Can you work these out from the model? Positions are in its coordinate system, mm. Give positions to 0.01 mm unless a question says otherwise; leave off trailing zeros. Answer as a JSON object with one key per item and string values.
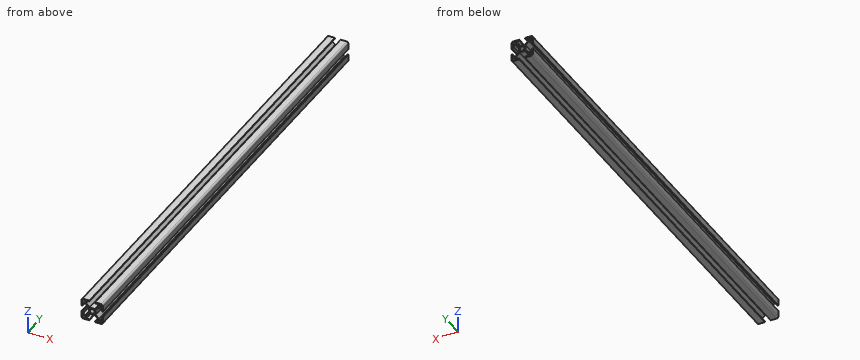
```python
from build123d import *

# Parameters (mm, degrees)
SKETCH_1_R      = 3.4
EXTRUDE_1_DEPTH = 650


with BuildPart() as part:
    # 草图1 → 凸台-拉伸1 (new body)
    with BuildSketch(Plane(origin=(0, 0, 0), x_dir=(1, 0, 0), z_dir=(0, 1, 0))):
        with BuildLine():
            Line((-4.1, 15), (-12.5, 15))
            ThreePointArc((-12.5, 15), (-14.267766953, 14.267766953), (-15, 12.5))
            Line((-15, 12.5), (-15, 4.1))
            Line((-15, 4.1), (-13.5, 4.1))
            Line((-13.5, 4.1), (-13.5, 8.4))
            Line((-13.5, 8.4), (-9.460660172, 8.4))
            Line((-9.460660172, 8.4), (-4.75, 3.689339828))
            Line((-4.75, 3.689339828), (-4.75, -3.689339828))
            Line((-4.75, -3.689339828), (-9.460660172, -8.4))
            Line((-9.460660172, -8.4), (-13.5, -8.4))
            Line((-13.5, -8.4), (-13.5, -4.1))
            Line((-13.5, -4.1), (-15, -4.1))
            Line((-15, -4.1), (-15, -12.5))
            ThreePointArc((-15, -12.5), (-14.267766953, -14.267766953), (-12.5, -15))
            Line((-12.5, -15), (-4.1, -15))
            Line((-4.1, -15), (-4.1, -13.5))
            Line((-4.1, -13.5), (-8.4, -13.5))
            Line((-8.4, -13.5), (-8.4, -9.460660172))
            Line((-8.4, -9.460660172), (-3.689339828, -4.75))
            Line((-3.689339828, -4.75), (3.689339828, -4.75))
            Line((3.689339828, -4.75), (8.4, -9.460660172))
            Line((8.4, -9.460660172), (8.4, -13.5))
            Line((8.4, -13.5), (4.1, -13.5))
            Line((4.1, -13.5), (4.1, -15))
            Line((4.1, -15), (12.5, -15))
            ThreePointArc((12.5, -15), (14.267766953, -14.267766953), (15, -12.5))
            Line((15, -12.5), (15, -4.1))
            Line((15, -4.1), (13.5, -4.1))
            Line((13.5, -4.1), (13.5, -8.4))
            Line((13.5, -8.4), (9.460660172, -8.4))
            Line((9.460660172, -8.4), (4.75, -3.689339828))
            Line((4.75, -3.689339828), (4.75, 3.689339828))
            Line((4.75, 3.689339828), (9.460660172, 8.4))
            Line((9.460660172, 8.4), (13.5, 8.4))
            Line((13.5, 8.4), (13.5, 4.1))
            Line((13.5, 4.1), (15, 4.1))
            Line((15, 4.1), (15, 12.5))
            ThreePointArc((15, 12.5), (14.267766953, 14.267766953), (12.5, 15))
            Line((12.5, 15), (4.1, 15))
            Line((4.1, 15), (4.1, 13.5))
            Line((4.1, 13.5), (8.4, 13.5))
            Line((8.4, 13.5), (8.4, 9.460660172))
            Line((8.4, 9.460660172), (3.689339828, 4.75))
            Line((3.689339828, 4.75), (-3.689339828, 4.75))
            Line((-3.689339828, 4.75), (-8.4, 9.460660172))
            Line((-8.4, 9.460660172), (-8.4, 13.5))
            Line((-8.4, 13.5), (-4.1, 13.5))
            Line((-4.1, 13.5), (-4.1, 15))
        make_face()
        with Locations(Location((0, 0, 0), (0, 0, 270))):
            Circle(SKETCH_1_R, mode=Mode.SUBTRACT)
        with BuildLine():
            Line((-10.7, 13.7), (-12.7, 13.7))
            ThreePointArc((-12.7, 13.7), (-13.407106781, 13.407106781), (-13.7, 12.7))
            Line((-13.7, 12.7), (-13.7, 10.7))
            ThreePointArc((-13.7, 10.7), (-13.407106781, 9.992893219), (-12.7, 9.7))
            Line((-12.7, 9.7), (-10.7, 9.7))
            ThreePointArc((-10.7, 9.7), (-9.992893219, 9.992893219), (-9.7, 10.7))
            Line((-9.7, 10.7), (-9.7, 12.7))
            ThreePointArc((-9.7, 12.7), (-9.992893219, 13.407106781), (-10.7, 13.7))
        make_face(mode=Mode.SUBTRACT)
        with BuildLine():
            Line((13.7, 10.7), (13.7, 12.7))
            ThreePointArc((13.7, 12.7), (13.407106781, 13.407106781), (12.7, 13.7))
            Line((12.7, 13.7), (10.7, 13.7))
            ThreePointArc((10.7, 13.7), (9.992893219, 13.407106781), (9.7, 12.7))
            Line((9.7, 12.7), (9.7, 10.7))
            ThreePointArc((9.7, 10.7), (9.992893219, 9.992893219), (10.7, 9.7))
            Line((10.7, 9.7), (12.7, 9.7))
            ThreePointArc((12.7, 9.7), (13.407106781, 9.992893219), (13.7, 10.7))
        make_face(mode=Mode.SUBTRACT)
        with BuildLine():
            Line((10.7, -13.7), (12.7, -13.7))
            ThreePointArc((12.7, -13.7), (13.407106781, -13.407106781), (13.7, -12.7))
            Line((13.7, -12.7), (13.7, -10.7))
            ThreePointArc((13.7, -10.7), (13.407106781, -9.992893219), (12.7, -9.7))
            Line((12.7, -9.7), (10.7, -9.7))
            ThreePointArc((10.7, -9.7), (9.992893219, -9.992893219), (9.7, -10.7))
            Line((9.7, -10.7), (9.7, -12.7))
            ThreePointArc((9.7, -12.7), (9.992893219, -13.407106781), (10.7, -13.7))
        make_face(mode=Mode.SUBTRACT)
        with BuildLine():
            Line((-13.7, -10.7), (-13.7, -12.7))
            ThreePointArc((-13.7, -12.7), (-13.407106781, -13.407106781), (-12.7, -13.7))
            Line((-12.7, -13.7), (-10.7, -13.7))
            ThreePointArc((-10.7, -13.7), (-9.992893219, -13.407106781), (-9.7, -12.7))
            Line((-9.7, -12.7), (-9.7, -10.7))
            ThreePointArc((-9.7, -10.7), (-9.992893219, -9.992893219), (-10.7, -9.7))
            Line((-10.7, -9.7), (-12.7, -9.7))
            ThreePointArc((-12.7, -9.7), (-13.407106781, -9.992893219), (-13.7, -10.7))
        make_face(mode=Mode.SUBTRACT)
    extrude(amount=EXTRUDE_1_DEPTH)


solid = part.part
```
1) I want a section at A-A on y = 61. Count the separate pieces of the cut face and the enclosed holes in it, and give its area (3 significant figures).
Results found:
{"separate pieces": "1", "enclosed holes": "5", "area": "249 mm²"}
2) I'm going to push flat-ended pins straight in: pin 1 Ø1.2 at (y, z) = (484, -14) entering from -X; pin 2 Ø2 at (x, y) = (0, 402.5) entering from +Z; pin 3 Ø1.6 at (x, y) = (-14, 397) entering from +Z. Where does each tip first touch, or does it pass through?
Results found:
{"pin 1": "stops at x = -14.83", "pin 2": "stops at z = 4.75", "pin 3": "stops at z = 14.9"}
3) I need wall thicknesses on L1, parallel to X at y = 312, z = 0; L2, parallel to Z at x = -12.25, y = 230.5; L3, parallel to X at y = 568, z = -10. Which ranges of each line are inside material? Lowest first, please.
Results found:
{"L1": "x = -4.75 to -3.4, 3.4 to 4.75", "L2": "z = -15 to -13.7, -9.7 to -8.4, 8.4 to 9.7, 13.7 to 15", "L3": "x = -15 to -13.41, -9.99 to -8.4, 8.4 to 9.99, 13.41 to 15"}
